Check sheet for the drawn part. Datum: minimum x, y, z corner. Units: mm. A direction names the side the tool comes from. Coordinates: 2 decimals unless noted, no trailing zeros. Loops run counter-clockwise (first coordinate to the right, second up) from the corner with the lowest first, then second, coordinate; pieces in that order, holes last.
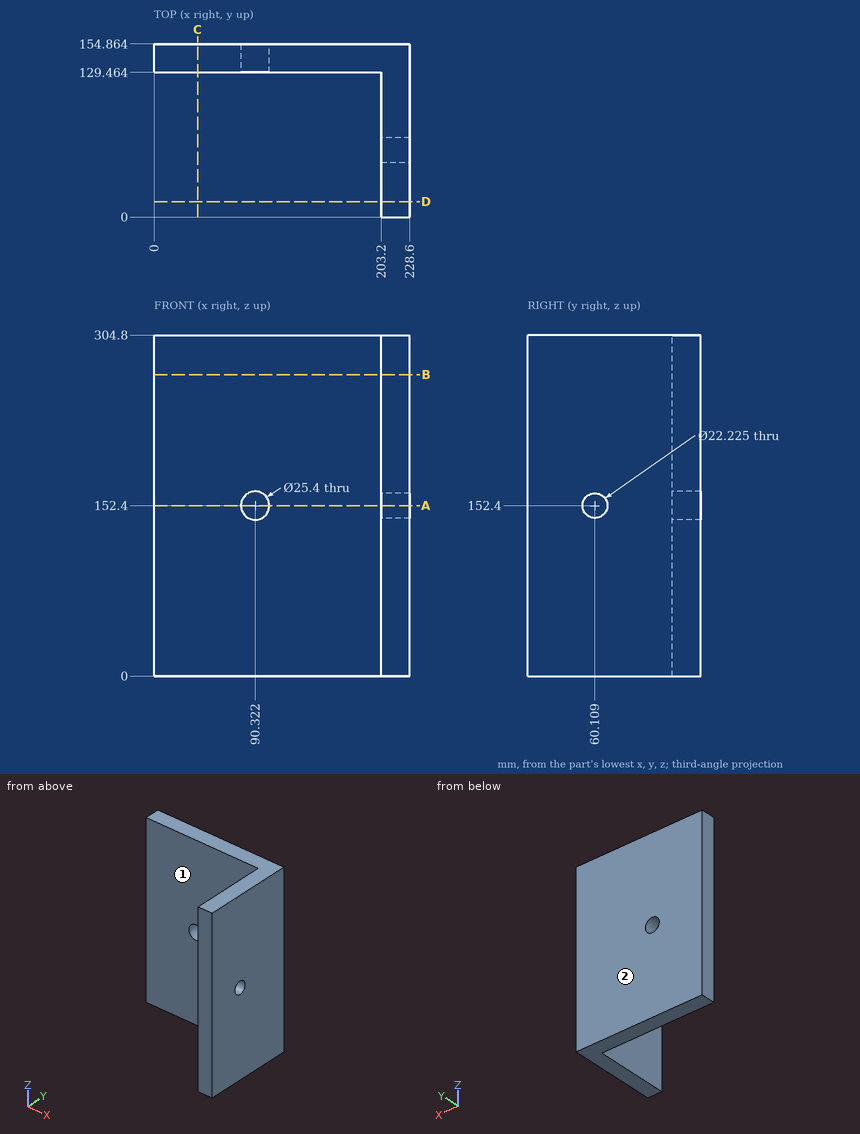
(1) Sectioned sample at A-A on z = 152.4. Record the cut outline in (x, y).
Findings:
outline: (0, 129.46) - (77.62, 129.46) - (77.62, 154.86) - (0, 154.86) - close; (103.02, 129.46) - (203.2, 129.46) - (203.2, 71.22) - (228.6, 71.22) - (228.6, 154.86) - (103.02, 154.86) - close; (203.2, 0) - (228.6, 0) - (228.6, 49) - (203.2, 49) - close
(2) Gauge pin test, flat ends, axial feed: pin 1 Ø6 at (y, z) = (60.5, 210) entering from -X; pin 2 Ø10 at (x, z) = (83.5, 267) entering from -Y. Record the tip position at first contact, or that the pin passes through.
Findings:
pin 1: stops at x = 203.2
pin 2: stops at y = 129.46
(3) Sectioned sample at D-D on y = 14. Record the cut outline in (x, z), and give its area (3 significant figures).
Findings:
outline: (203.2, 0) - (228.6, 0) - (228.6, 304.8) - (203.2, 304.8) - close
area: 7,740 mm2
(4) Sectioned sample at C-C on x = 39. Record the cut outline in (y, z), and give its area (3 significant figures).
Findings:
outline: (129.46, 0) - (154.86, 0) - (154.86, 304.8) - (129.46, 304.8) - close
area: 7,740 mm2
(5) Access from +Z, -Z, +X, -X, +Y, -Y to the whole of each face (thin tool, end or side, straight path). Record for the marked faces 1 and 2.
Findings:
face 1: +Z, -Z, -X, -Y
face 2: +Z, -Z, +X, -X, +Y
(6) Scan lines: L1, parallel to Y at x = 218, z = 152 (1 decimal); L2, parallel to Y at x = 152.5, z = 166.5; L3, parallel to X at y = 44, z = 188.5. Record each from-to range of solid material in increasing order.
Findings:
L1: y = 0 to 49, 71.2 to 154.9
L2: y = 129.46 to 154.86
L3: x = 203.2 to 228.6
(7) Sectioned sample at B-B on z = 269.5. Record the cut outline in (x, y).
Findings:
outline: (0, 129.46) - (203.2, 129.46) - (203.2, 0) - (228.6, 0) - (228.6, 154.86) - (0, 154.86) - close
